```python
from build123d import *

# Parameters (mm, degrees)
SKETCH1_W                 = 67.5
SKETCH1_H                 = 50
BOSS_EXTRUDE1_DEPTH       = 6.35
EDGE_FLANGE1_DEPTH        = 50
EDGE_FLANGE1_START        = -6.35
EDGE_FLANGE1_FLAT_DEPTH   = 6.35
EDGE_FLANGE1_BEND_DEPTH   = 50
EDGE_FLANGE1_FLAT_2_DEPTH = 6.35
CUT_EXTRUDE1_DEPTH        = 141.387472732
CUT_EXTRUDE3_DEPTH        = 3.175
SKETCH16_R                = 2.54
CUT_EXTRUDE4_DEPTH        = 122.784135358
SKETCH17_R                = 6.35
CUT_EXTRUDE5_DEPTH        = 122.784135358
SKETCH18_R                = 25.4
CUT_EXTRUDE6_DEPTH        = 3.175
CUT_EXTRUDE7_START        = -3.175
SKETCH19_R                = 25.4
CUT_EXTRUDE7_DEPTH        = 3.175
SKETCH20_R                = 2.54
CUT_EXTRUDE8_DEPTH        = 139.460655513


# Sheet-metal steps are written as plain solids
with BuildPart() as part:
    # Sketch1 → Boss-Extrude1 (new body)
    with BuildSketch(Plane(origin=(0, 0, 0), x_dir=(1, 0, 0), z_dir=(0, 1, 0))):
        Rectangle(SKETCH1_W, SKETCH1_H)
    extrude(amount=BOSS_EXTRUDE1_DEPTH)

    # Edge-Flange1 bend section (across the edge) → Edge-Flange1 (add)
    with BuildSketch(Plane(origin=(36.75, 0, -25), x_dir=(-1, 0, 0), z_dir=(0, 0, 1))):
        with BuildLine():
            Line((-6.35, 3), (0, 3))
            ThreePointArc((0, 3), (0.878679656, 0.878679656), (3, 0))
            Line((3, 0), (3, -6.35))
            ThreePointArc((3, -6.35), (-3.611448404, -3.611448404), (-6.35, 3))
        make_face()
    extrude(amount=EDGE_FLANGE1_DEPTH)

    # Edge-Flange1 profile (on flange) → Edge-Flange1 flat (add)
    with BuildSketch(Plane(origin=(36.75, 0, 0), x_dir=(0, 0, -1), z_dir=(-1, 0, 0)).offset(EDGE_FLANGE1_START)):
        with BuildLine():
            ThreePointArc((25, 82.95), (0, 107.95), (-25, 82.95))
            Line((-25, 82.95), (-25, 3))
            Line((-25, 3), (25, 3))
            Line((25, 3), (25, 82.95))
        make_face()
    extrude(amount=EDGE_FLANGE1_FLAT_DEPTH)

    # Edge-Flange1 bend section 2 (across the edge) → Edge-Flange1 bend (add)
    with BuildSketch(Plane(origin=(-36.75, 0, 25), x_dir=(1, 0, 0), z_dir=(0, 0, -1))):
        with BuildLine():
            Line((-6.35, 3), (0, 3))
            ThreePointArc((0, 3), (0.878679656, 0.878679656), (3, 0))
            Line((3, 0), (3, -6.35))
            ThreePointArc((3, -6.35), (-3.611448404, -3.611448404), (-6.35, 3))
        make_face()
    extrude(amount=EDGE_FLANGE1_BEND_DEPTH)

    # Edge-Flange1 profile 2 (on flange) → Edge-Flange1 flat 2 (add)
    with BuildSketch(Plane(origin=(-36.75, 0, 0), x_dir=(0, 0, 1), z_dir=(1, 0, 0)).offset(EDGE_FLANGE1_START)):
        with BuildLine():
            ThreePointArc((25, 82.95), (0, 107.95), (-25, 82.95))
            Line((-25, 82.95), (-25, 3))
            Line((-25, 3), (25, 3))
            Line((25, 3), (25, 82.95))
        make_face()
    extrude(amount=EDGE_FLANGE1_FLAT_2_DEPTH)

    # Sketch13 → Cut-Extrude1 (cut, through all)
    with BuildSketch(Plane.ZY.offset(43.1)):
        with BuildLine():
            Line((9.797958971, -87.95), (25, -87.95))
            Line((25, -87.95), (25, -77.95))
            Line((25, -77.95), (9.797958971, -77.95))
            ThreePointArc((9.797958971, -77.95), (-11, -82.95), (9.797958971, -87.95))
        make_face()
    extrude(amount=-CUT_EXTRUDE1_DEPTH, mode=Mode.SUBTRACT)

    # Sketch15 → Cut-Extrude3 (cut)
    with BuildSketch(Plane(origin=(0, 6.35, 0), x_dir=(1, 0, 0), z_dir=(0, 1, 0))):
        with BuildLine():
            Line((-11.25, 22.225), (11.25, 22.225))
            ThreePointArc((11.25, 22.225), (33.475, 0), (11.25, -22.225))
            Line((11.25, -22.225), (-11.25, -22.225))
            ThreePointArc((-11.25, -22.225), (-33.475, 0), (-11.25, 22.225))
        make_face()
    extrude(amount=-CUT_EXTRUDE3_DEPTH, mode=Mode.SUBTRACT)

    # Sketch16 → Cut-Extrude4 (cut, through all)
    with BuildSketch(Plane(origin=(0, 3.175, 0), x_dir=(1, 0, 0), z_dir=(0, 1, 0))):
        with Locations(Location((-21.036441357, -11.663026646, 0), (0, 0, 270))):
            Circle(SKETCH16_R)
        with Locations(Location((-21.036441357, 11.663026646, 0), (0, 0, 270))):
            Circle(SKETCH16_R)
        with Locations(Location((21.036441357, 11.663026646, 0), (0, 0, 270))):
            Circle(SKETCH16_R)
        with Locations(Location((21.036441357, -11.663026646, 0), (0, 0, 270))):
            Circle(SKETCH16_R)
    extrude(amount=-CUT_EXTRUDE4_DEPTH, mode=Mode.SUBTRACT)

    # Sketch17 → Cut-Extrude5 (cut, through all)
    with BuildSketch(Plane(origin=(0, 3.175, 0), x_dir=(1, 0, 0), z_dir=(0, 1, 0))):
        with Locations(Location((0, 0, 0), (0, 0, 270))):
            Circle(SKETCH17_R)
    extrude(amount=-CUT_EXTRUDE5_DEPTH, mode=Mode.SUBTRACT)

    # Sketch18 → Cut-Extrude6 (cut)
    with BuildSketch(Plane.ZY.offset(43.1)):
        with Locations((0, -82.95)):
            Circle(SKETCH18_R)
    extrude(amount=-CUT_EXTRUDE6_DEPTH, mode=Mode.SUBTRACT)

    # Sketch19 → Cut-Extrude7 (cut)
    with BuildSketch(Plane(origin=(43.1, 0, 0), x_dir=(0, 0, -1), z_dir=(1, 0, 0)).offset(CUT_EXTRUDE7_START)):
        with Locations((0, -82.95)):
            Circle(SKETCH19_R)
    extrude(amount=CUT_EXTRUDE7_DEPTH, mode=Mode.SUBTRACT)

    # Sketch20 → Cut-Extrude8 (cut, through all)
    with BuildSketch(Plane(origin=(39.925, 0, 0), x_dir=(0, 0, -1), z_dir=(1, 0, 0))):
        with Locations(Location((18.4, -82.95, 0), (0, 0, 150.134638176))):
            Circle(SKETCH20_R)
        with Locations(Location((5.685912696, -100.4494399, 0), (0, 0, 90))):
            Circle(SKETCH20_R)
        with Locations(Location((-14.885912696, -93.765248642, 0), (0, 0, 90))):
            Circle(SKETCH20_R)
        with Locations(Location((-14.885912696, -72.134751358, 0), (0, 0, 90))):
            Circle(SKETCH20_R)
        with Locations(Location((5.685912696, -65.4505601, 0), (0, 0, 90))):
            Circle(SKETCH20_R)
    extrude(amount=-CUT_EXTRUDE8_DEPTH, mode=Mode.SUBTRACT)


solid = part.part
```
Here's how the part is built. I have some questions about the finished solid (model axes, mm). A direction names the side the tool comes from. Coordinates: 2 decimals unless noted, no trailing zeros. Write each loop counter-clockwise with the first axis right and the second up, starting at its lowest first coordinate (ties: lowest second). Pieces come first, ordered by that corner, then holes. Notation, with made-up numbers: M -7,-16 L 10,-16 A22 ccw 10,7 Z; hole C 6.25,20 d6. An arc over 180 degrees is marked long. Answer as CSV lines item,"result". Start each with the question number.
Q1. Suppose I cut it at B-B, the plane y = -55. List the corners of the cut face in (x, z) for me, then the cut area to 3 significant figures.
Q2. Suppose I cut it at C-C, the plane z = -19. List the corners of the cut face in (x, y) for me (3 decimals).
Q3. I need wall thicknesses on probe 1 along X at (y, z) = (-19.5, -3); probe 2 along X at (y, z) = (-63.5, 1) (3 decimals); probe 3 along Z at (x, y) = (39.2, -82.95). Which ranges of each line are inside material? Lowest first, please. Write a range as [from, to].
Q4. Will these pins go through, and if not, where does the flat tip stop? pin 1 Ø6.5 at (y, z) = (-72.13, 14.89) entering from +X (3 decimals); pin 2 Ø4.5 at (y, z) = (-100.45, -5.69) entering from -X; pin 3 Ø3 at (x, z) = (-40.5, 20.5) entering from -Y; pin 4 Ø1 at (x, z) = (-27, 15) entering from -Y.
Q5. Suppose I cut it at A-A, the plane x = 0. List the corners of the cut face in (y, z) for me (3 decimals), then the cut area to 3 significant figures.
Q6. Suppose I cut it at D-D, the plane z = 0. State how many separate pieces and enclosed holes the cut face has, then the cut area to 3 significant figures.
Q7. If we mould it in two halves opening along X, with no side actions, what happens to faces 1 (the flat face through (-38, -87.95, 17)), 2 (the flat face through (39.925, -88, -11)), 3 (the flat face through (-7, 3.175, 0))? For each: pulls with the +X half, pulls with the -X half, needs draft (parallel to the pull), parting line crosses it, or undercut.
Q8. For faces 4 (the cylindrical face through (22.75, 1.61, 9.79)), 5 (the cylindrical face through (-41.53, -57.55, 0.23)), 6 (the flat face through (-38, -77.95, 18)), which set-ups out of +Z, -Z, +X, -X, +Y, -Y let a thin tool reach every point of the face, with its end or its side?
Entries:
1,outline,"M -43.1,-25 L -36.75,-25 L -36.75,25 L -43.1,25 Z; M 36.75,-25 L 43.1,-25 L 43.1,25 L 36.75,25 Z"
1,area,"635 mm²"
2,outline,"M -43.1,-66.093 L -39.925,-66.093 L -39.925,-80.482 L -36.75,-80.482 L -36.75,-3 A3 cw -33.75,0 L 33.75,0 A3 cw 36.75,-3 L 36.75,-80.482 L 39.925,-80.482 L 39.925,-66.093 L 43.1,-66.093 L 43.1,-3 A9.35 ccw 33.75,6.35 L 22.78,6.35 L 22.78,3.175 L -22.78,3.175 L -22.78,6.35 L -33.75,6.35 A9.35 ccw -43.1,-3 Z; M -39.925,-99.198 L -36.75,-99.198 L -36.75,-85.418 L -39.925,-85.418 Z; M 36.75,-99.198 L 39.925,-99.198 L 39.925,-85.418 L 36.75,-85.418 Z"
3,probe 1,"x = [-43.1, -36.75], [36.75, 43.1]"
3,probe 2,"x = [-39.925, -36.75], [36.75, 39.925]"
3,probe 3,"z = [-25, -20.94], [-15.86, -11]"
4,pin 1,"stops at x = 39.925"
4,pin 2,"passes through"
4,pin 3,"stops at y = -99.06"
4,pin 4,"stops at y = 0"
5,outline,"M 0,-25 L 6.35,-25 L 6.35,-22.225 L 3.175,-22.225 L 3.175,-6.35 L 0,-6.35 Z; M 0,6.35 L 3.175,6.35 L 3.175,22.225 L 6.35,22.225 L 6.35,25 L 0,25 Z"
5,area,"136 mm²"
6,separate pieces,"4"
6,enclosed holes,"0"
6,area,"1,170 mm²"
7,face 1,"needs draft"
7,face 2,"pulls with the +X half"
7,face 3,"undercut"
8,face 4,"+Y, -Y"
8,face 5,"-X, -Y"
8,face 6,"+Z, +X, -X"
